Drawing for the job (mm, zero at the part's lowest x, y, z). Give positions to 0.01 mm unless a question says otherwise; leave off trailing zeros. Order: outer loops, then holes, each group sorted by start corner. A loop starts at its lowest first (then second) coordinate and runs counter-clockwise, first axis right, second up. Notation, with made-up numbers: M -28.5,80 L 1.5,80 A27 cw 1.5,109 Z; hole C 9.5,64.5 d3. An arc over 180 degrees is marked long. Answer as a JSON object with one key per item and string values.
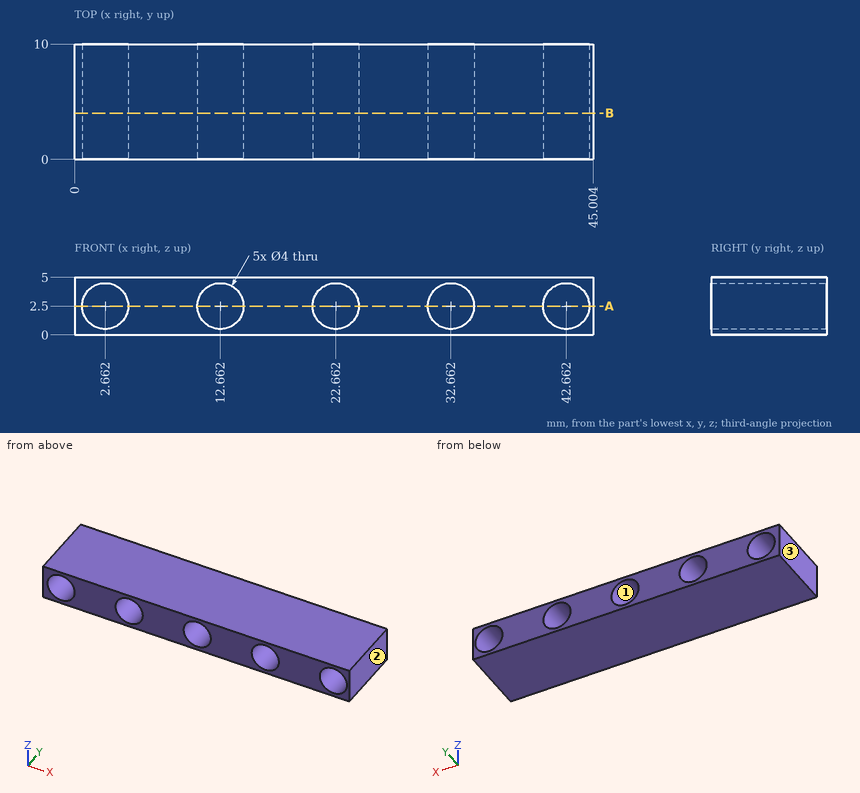
1. Cut at A-A on z = 2.5. Give the cut face in (x, y).
Worked answers:
{"outline": "M 0,0 L 0.66,0 L 0.66,10 L 0,10 Z; M 4.66,0 L 10.66,0 L 10.66,10 L 4.66,10 Z; M 14.66,0 L 20.66,0 L 20.66,10 L 14.66,10 Z; M 24.66,0 L 30.66,0 L 30.66,10 L 24.66,10 Z; M 34.66,0 L 40.66,0 L 40.66,10 L 34.66,10 Z; M 44.66,0 L 45,0 L 45,10 L 44.66,10 Z"}
2. Cut at B-B on y = 4. Give the cut face in (x, z).
Worked answers:
{"outline": "M 0,0 L 45,0 L 45,5 L 0,5 Z; hole C 2.66,2.5 d4; hole C 12.66,2.5 d4; hole C 22.66,2.5 d4; hole C 32.66,2.5 d4; hole C 42.66,2.5 d4"}
3. Probe line 1 along X through (y, z) = (6.25, 2.5); line 2 along Z through (x, y) = (32.5, 6.75); line 3 along X through (y, z) = (7.5, 3.15). List the from-to ranges inside material, lowest first.
Worked answers:
{"line 1": "x = 0 to 0.66, 4.66 to 10.66, 14.66 to 20.66, 24.66 to 30.66, 34.66 to 40.66, 44.66 to 45", "line 2": "z = 0 to 0.51, 4.49 to 5", "line 3": "x = 0 to 0.77, 4.55 to 10.77, 14.55 to 20.77, 24.55 to 30.77, 34.55 to 40.77, 44.55 to 45"}
4. Two-plate mould, pull along X, no slides. Class the marked faces 1, 2 and 3: +X half, -X half, draft (parallel to the pull), parting line (faces both ways), or undercut.
Worked answers:
{"face 1": "undercut", "face 2": "+X half", "face 3": "-X half"}
